```python
from build123d import *

# Parameters (mm, degrees)
SKETCH215_R     = 3
PAD127051_DEPTH = 2
PAD127048_DEPTH = 3
PAD127047_DEPTH = 3
SKETCH209_R     = 3.5
PAD127045_DEPTH = 30
SKETCH210_R     = 4.25
PAD127046_DEPTH = 3
SKETCH216_R     = 3
PAD127052_DEPTH = 2
SKETCH208_W     = 10
SKETCH208_H     = 13
PAD127044_DEPTH = 14
SKETCH207_R     = 1.4
PAD127043_DEPTH = 3


with BuildPart() as countersinktop:
    # Sketch215 → Pad127051 (new body)
    with BuildSketch(Plane(origin=(50, 160, 5), x_dir=(1, 0, 0), z_dir=(0, 0, 1))):
        Circle(SKETCH215_R)
    extrude(amount=-PAD127051_DEPTH)


with BuildPart() as steeringrodcutoutbottom:
    # Sketch212 → Pad127048 (new body)
    with BuildSketch(Plane(origin=(50, 160, -5), x_dir=(1, 0, 0), z_dir=(0, 0, 1))):
        with BuildLine():
            Line((9, 3.875), (3.392179, 3.875))
            ThreePointArc((3.392179, 3.875), (0, 5.15), (-3.392179, 3.875))
            Line((-3.392179, 3.875), (-8, 3.875))
            Line((-8, 3.875), (-8, -3.875))
            Line((-8, -3.875), (-3.392179, -3.875))
            ThreePointArc((-3.392179, -3.875), (0, -5.15), (3.392179, -3.875))
            Line((3.392179, -3.875), (9, -3.875))
            Line((9, -2.5), (9, -3.875))
            Line((12, -2.5), (9, -2.5))
            Line((12, 2.5), (12, -2.5))
            Line((9, 2.5), (12, 2.5))
            Line((9, 3.875), (9, 2.5))
        make_face()
    extrude(amount=-PAD127048_DEPTH)


with BuildPart() as steeringrodcutouttop:
    # Sketch211 → Pad127047 (new body)
    with BuildSketch(Plane(origin=(50, 160, 5), x_dir=(1, 0, 0), z_dir=(0, 0, 1))):
        with BuildLine():
            Line((9, 3.875), (3.392179, 3.875))
            ThreePointArc((3.392179, 3.875), (0, 5.15), (-3.392179, 3.875))
            Line((-3.392179, 3.875), (-8, 3.875))
            Line((-8, 3.875), (-8, -3.875))
            Line((-8, -3.875), (-3.392179, -3.875))
            ThreePointArc((-3.392179, -3.875), (0, -5.15), (3.392179, -3.875))
            Line((3.392179, -3.875), (9, -3.875))
            Line((9, -2.5), (9, -3.875))
            Line((12, -2.5), (9, -2.5))
            Line((12, 2.5), (12, -2.5))
            Line((9, 2.5), (12, 2.5))
            Line((9, 3.875), (9, 2.5))
        make_face()
    extrude(amount=PAD127047_DEPTH)


with BuildPart() as axlecutout:
    # Sketch209 → Pad127045 (new body)
    with BuildSketch(Plane(origin=(59, 160, 0), x_dir=(0, 1, 0), z_dir=(1, 0, 0))):
        Circle(SKETCH209_R)
    extrude(amount=-PAD127045_DEPTH)


with BuildPart() as bearingcutout:
    # Sketch210 → Pad127046 (new body)
    with BuildSketch(Plane(origin=(45, 160, 0), x_dir=(0, 1, 0), z_dir=(1, 0, 0))):
        Circle(SKETCH210_R)
    extrude(amount=PAD127046_DEPTH)


with BuildPart() as cutouts:
    # Sketch216 → Pad127052 (new body)
    with BuildSketch(Plane(origin=(50, 160, -5), x_dir=(1, 0, 0), z_dir=(0, 0, 1))):
        Circle(SKETCH216_R)
    extrude(amount=PAD127052_DEPTH)

    # Fusion004020029: union CountersinkTop, SteeringRodCutoutBottom, SteeringRodCutoutTop, AxleCutout, BearingCutout
    add(countersinktop.part)
    add(steeringrodcutoutbottom.part)
    add(steeringrodcutouttop.part)
    add(axlecutout.part)
    add(bearingcutout.part)


with BuildPart() as mainbody:
    # Sketch208 → Pad127044 (new body)
    with BuildSketch(Plane(origin=(59, 160, 0), x_dir=(0, 1, 0), z_dir=(1, 0, 0))):
        Rectangle(SKETCH208_W, SKETCH208_H)
    extrude(amount=-PAD127044_DEPTH)


with BuildPart() as steeringcolumn:
    # Sketch207 → Pad127043 (new body)
    with BuildSketch(Plane(origin=(59, 160, 0), x_dir=(0, 1, 0), z_dir=(1, 0, 0))):
        with BuildLine():
            ThreePointArc((9.118035, 1.763933), (10.236068, 5.118034), (6.881967, 6.236069))
            Line((6.881967, 6.236069), (-9.118034, -1.763932))
            ThreePointArc((-9.118034, -1.763932), (-10.236068, -5.118034), (-6.881966, -6.236068))
            Line((-6.881966, -6.236068), (9.118035, 1.763933))
        make_face()
        with Locations((8, 4)):
            Circle(SKETCH207_R, mode=Mode.SUBTRACT)
        with Locations((-8, -4)):
            Circle(SKETCH207_R, mode=Mode.SUBTRACT)
    extrude(amount=-PAD127043_DEPTH)

    # Fusion004020028: union MainBody
    add(mainbody.part)

    # Cut007019028: cut cutouts
    add(cutouts.part, mode=Mode.SUBTRACT)


solid = steeringcolumn.part
```
Model file for the job. Use its own axes, mm. A direction names the side the tool comes from. Coordinates: 2 decimals unless noted, no trailing zeros. Loops run counter-clockwise (first coordinate to the right, second up) from the corner with the lowest first, then second, coordinate; pieces in that order, holes last. Notation, with made-up numbers: M 16.5,54 L 64.5,54 A23 ccw 64.5,72 Z; hole C 79.5,37.5 d4. An arc over 180 degrees is marked long. Use CSV: the item, a comma, the result in double quotes. Start each with the question number.
1. Band-saw the part on B-B, the plane x = 58. List the corners of the cut face in (y, z) (3 decimals), then the cut area to 3 significant figures.
2. Flat gauge pins, fed straight in: pin 1 (1.6 mm diameter, centred on x = 56.5, z = -6, fed in from -Y); pin 2 (1.6 mm diameter, centred on x = 46, z = 5.5, fed in from +Y); pin 3 (5 mm diameter, centred on x = 50, y = 160, fed in from +Z). Where does each tip first touch, or does it go through?
3. Band-saw the part on C-C, the plane z = -4. List the corners of the cut face in (x, y).
4. Band-saw the part on D-D, the plane x = 50. List the corners of the cut face in (y, z).
5. Two-plate mould, pull along X, no slides. Class faces 4 (the cylindrical face through (47.604, 155.441, 5.74)), 5 (the flat face through (52, 165, 0)), 6 (the flat face through (56, 166, 3)): pulls with the +X half, pulls with the -X half, needs draft (parallel to the pull), parting line crosses it, or undercut.
6. Tool access for faces 1 (the cylindrical face through (47.635, 164.575, 5.74)), 2 (the cylindrical face through (52.86, 160.9, -4.24)), 3 (the flat face through (56, 163.875, -6)): list every direction of +Z, -Z, +X, -X, +Y, -Y with a clear straight run to the whole face (end or side of a thin tool).
7. Probe probe 1 along Y at (x, z) = (46.5, -5.25) (3 decimals); probe 2 along Z at (x, y) = (54.5, 160); probe 3 along Y at (x, z) = (50, 4.15). List the from-to ranges inside material, lowest first. Write a range as [from, to].
8. Band-saw the part on A-A, the plane y = 160. List the corners of the cut face in (x, z).
Entries:
1,outline,"M 150.882,-1.764 A2.5 ccw 153.118,-6.236 L 155,-5.295 L 155,-6.5 L 156.125,-6.5 L 156.125,-5 L 163.875,-5 L 163.875,-6.5 L 165,-6.5 L 165,-0.295 L 169.118,1.764 A2.5 ccw 166.882,6.236 L 165,5.295 L 165,6.5 L 163.875,6.5 L 163.875,5 L 156.125,5 L 156.125,6.5 L 155,6.5 L 155,0.295 Z; hole C 152,-4 d2.8; hole C 160,0 d7; hole C 168,4 d2.8"
1,area,"109 mm2"
2,pin 1,"stops at y = 149.81"
2,pin 2,"stops at y = 165"
2,pin 3,"stops at z = 3"
3,outline,"M 45,155 L 56,155 L 56,153.4 L 59,153.4 L 59,165 L 45,165 L 45,161.44 L 47.37,161.44 A3 cw long 47.37,158.56 L 45,158.56 Z; M 56,149.5 L 59,149.5 L 59,150.6 L 56,150.6 Z"
4,outline,"M 155,-5 L 157,-5 L 157,-3 L 158.2,-3 A3.5 cw 158.2,3 L 157,3 L 157,5 L 155,5 Z; M 161.8,-3 L 163,-3 L 163,-5 L 165,-5 L 165,5 L 163,5 L 163,3 L 161.8,3 A3.5 cw Z"
5,face 4,"undercut"
5,face 5,"needs draft"
5,face 6,"pulls with the -X half"
6,face 1,"+Z"
6,face 2,"-Z"
6,face 3,"-Z, +X, -X"
7,probe 1,"y = [155, 156.125], [163.875, 165]"
7,probe 2,"z = [-5, -3.5], [3.5, 5]"
7,probe 3,"y = [155, 157], [163, 165]"
8,outline,"M 45,-5 L 47,-5 L 47,-4.25 L 45,-4.25 Z; M 45,4.25 L 47,4.25 L 47,5 L 45,5 Z; M 53,-5 L 59,-5 L 59,-3.5 L 53,-3.5 Z; M 53,3.5 L 59,3.5 L 59,5 L 53,5 Z"
